Build history of the part. All positions in model axes, mm. Face numbers are marked on the shaded views. A direction names the side the tool comes from. Round coordinates to 2 decimals unless told otherwise and drop trailing zeros. Order: outer loops, then holes, each group sorted by start corner. A loop starts at its lowest first (then second) coordinate and runs counter-clockwise, first axis right, second up. Notation, with made-up numbers: M -30,26 L 23,26 A29 cw 23,59 Z; hole C 44,38 d3. An arc over 180 degrees is marked long. One line per item, written item: value. Start each with the question number.
Item 1: Tool access for the marked faces 1, 2 and 3: list every direction of +Z, -Z, +X, -X, +Y, -Y with a clear straight run to the whole face (end or side of a thin tool).
Item 2: Band-saw the part on A-A, the plane z = -8. Write the cut outline in (x, y).
Item 3: Pin check, flat tips, straight feed: pin 1 (6 mm diameter, centred on y = -4, z = -15.5, fed in from -X); pin 2 (4 mm diameter, centred on x = -2, y = 0.5, fed in from -Z); pin 3 (3 mm diameter, centred on y = 4, z = -8, fed in from -X). Stop position of each tip, or through.
Item 4: Probe L1, parallel to X at y = 0, z = -8.25; L2, parallel to Z at x = 2.5, y = 6.5; L3, parallel to Y at x = 2.25, z = 3. List the from-to ranges inside material, lowest first.
Item 5: Band-saw the part on C-C, the plane y = 0. Write the cut outline in (x, z).
Item 6: Band-saw the part on D-D, the plane z = -17.5. Write the cut outline in (x, y), then the cut area to 3 significant figures.
Item 7: Two-plate mould, pull along Y, no slides. Class the marked faces 4, 5 and 6: +Y half, -Y half, draft (parallel to the pull), parting line (faces both ways), or undercut.
Item 8: Band-saw the part on B-B, the plane x = 0. Write the cut outline in (y, z), then the cut area to 3 significant figures.
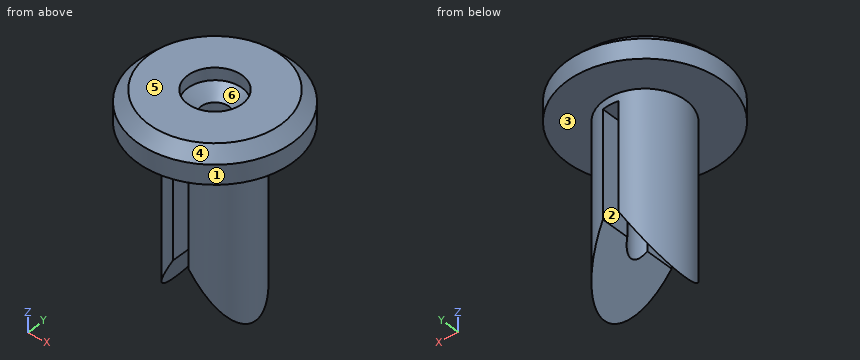
```python
from build123d import *

# Parameters (mm, degrees)
SKETCH002_W  = 2
SKETCH002_H  = 25
PAD001_DEPTH = 15
PAD_DEPTH    = 7.5


with BuildPart() as pad001:
    # Sketch002 → Pad001 (new body, symmetric)
    with BuildSketch(Plane.XZ):
        with Locations((0, -13.5)):
            Rectangle(SKETCH002_W, SKETCH002_H)
    extrude(amount=PAD001_DEPTH, both=True)


with BuildPart() as pad:
    # Sketch001 → Pad (new body, symmetric)
    with BuildSketch(Plane.XZ):
        Polygon((8, -26.856406), (0, -13), (-8, -26.856406), align=None)
    extrude(amount=PAD_DEPTH, both=True)


with BuildPart() as cut001:
    # Sketch → Revolution (revolve)
    with BuildSketch(Plane.XZ):
        Polygon((3.5, 4), (8.5, 4), (10, 2.5), (10, 0), (5.25, 0), (5.25, -23), (1.8, -23), (1.8, 1), (3.5, 2.426469), align=None)
    revolve(axis=Axis((0, 0, 0), (0, 0, 1)))

    # Cut: cut Pad
    add(pad.part, mode=Mode.SUBTRACT)

    # Cut001: cut Pad001
    add(pad001.part, mode=Mode.SUBTRACT)


solid = cut001.part
```
Output:
1. face 1: +Z, -Z
1. face 2: -Z, +Y, -Y
1. face 3: -Z
2. outline: M -1,-5.15 L -1,-1.5 A1.8 cw -1,1.5 L -1,5.15 A5.25 ccw Z; M 1,-5.15 A5.25 ccw 1,5.15 L 1,1.5 A1.8 cw 1,-1.5 Z
3. pin 1: stops at x = -5.15
3. pin 2: stops at z = -19.93
3. pin 3: stops at x = -4.62
4. L1: x = -5.25 to -1.8, 1.8 to 5.25
4. L2: z = 0 to 4
4. L3: y = -9.23 to -2.68, 2.68 to 9.23
5. outline: M -10,0 L -5.25,0 L -5.25,-22.09 L -1.8,-16.12 L -1.8,1 L -3.5,2.43 L -3.5,4 L -8.5,4 L -10,2.5 Z; M 1.8,-16.12 L 5.25,-22.09 L 5.25,0 L 10,0 L 10,2.5 L 8.5,4 L 3.5,4 L 3.5,2.43 L 1.8,1 Z
6. outline: M -2.6,-4.56 L -2.6,4.56 A5.25 ccw Z; M 2.6,-4.56 A5.25 ccw 2.6,4.56 Z
6. area: 34.3 mm²
7. face 4: parting line
7. face 5: draft
7. face 6: undercut
8. outline: M -10,0 L -5.25,0 L -5.25,-1 L -1.8,-1 L -1.8,1 L -3.5,2.43 L -3.5,4 L -8.5,4 L -10,2.5 Z; M 1.8,-1 L 5.25,-1 L 5.25,0 L 10,0 L 10,2.5 L 8.5,4 L 3.5,4 L 3.5,2.43 L 1.8,1 Z
8. area: 62.5 mm²
